Here's how the part is built. I have some questions about the finished solid (model axes, mm). A direction names the side the tool comes from. Coordinates: 2 decimals unless noted, no trailing zeros. Order: outer loops, then holes, each group sorted by start corner. A loop starts at its lowest first (then second) coordinate and runs counter-clockwise, first axis right, second up.
```python
from build123d import *

# Parameters (mm, degrees)
SKETCH1_W           = 12.25
SKETCH1_H           = 14.6
BOSS_EXTRUDE1_DEPTH = 13.13
CUT_EXTRUDE1_DEPTH  = 12.07
SKETCH4_W           = 10.22
SKETCH4_H           = 1.85
CUT_EXTRUDE3_DEPTH  = 10.5
CUT_EXTRUDE4_REACH  = 18.224
SKETCH5_W           = 0.518
SKETCH5_H           = 6.3
SKETCH6_W           = 9.9
SKETCH6_H           = 3.6
CUT_EXTRUDE5_DEPTH  = 1.9
SKETCH10_W          = 5.64
SKETCH10_H          = 2.85
CUT_EXTRUDE7_DEPTH  = 2.13
SKETCH11_W          = 9.9
SKETCH11_H          = 0.75
CUT_EXTRUDE8_DEPTH  = 15.728154161
SKETCH12_R          = 1
BOSS_EXTRUDE2_DEPTH = 2.9
FILLET1_R           = 0.25
SKETCH15_W          = 0.5
SKETCH15_H          = 0.5
BOSS_EXTRUDE3_DEPTH = 3.7
CHAMFER1_SIZE       = 0.05
SKETCH16_W          = 9.9
SKETCH16_H          = 0.6
BOSS_EXTRUDE4_DEPTH = 0.75
SKETCH17_W          = 0.518
SKETCH17_H          = 6.3
SKETCH17_W_2        = 10.25
SKETCH17_H_2        = 1.85
BOSS_EXTRUDE5_DEPTH = 2
SKETCH18_W          = 1.15
SKETCH18_H          = 10.25
BOSS_EXTRUDE6_DEPTH = 1


with BuildPart() as part:
    # Sketch1 → Boss-Extrude1 (new body)
    with BuildSketch(Plane.XY):
        Rectangle(SKETCH1_W, SKETCH1_H)
    extrude(amount=BOSS_EXTRUDE1_DEPTH)

    # Sketch2 → Cut-Extrude1 (cut)
    with BuildSketch(Plane.XY.offset(13.13)):
        Polygon((3.28, 3.2), (3.28, 4.75), (1.915, 4.75), (1.915, 6.55), (-1.915, 6.55), (-1.915, 4.75), (-3.28, 4.75), (-3.28, 3.2), (-4.95, 3.2), (-4.95, -3.7), (4.95, -3.7), (4.95, 3.2), align=None)
    extrude(amount=-CUT_EXTRUDE1_DEPTH, mode=Mode.SUBTRACT)

    # Sketch4 → Cut-Extrude3 (cut)
    with BuildSketch(Plane(origin=(0, 0, 0), x_dir=(-1, 0, 0), z_dir=(0, 0, -1))):
        with Locations((0, 5.375)):
            Rectangle(SKETCH4_W, SKETCH4_H)
    extrude(amount=-CUT_EXTRUDE3_DEPTH, mode=Mode.SUBTRACT)

    # Sketch5 → Cut-Extrude4 (cut, up to next)
    with BuildSketch(Plane(origin=(0, 0, 0), x_dir=(-1, 0, 0), z_dir=(0, 0, -1)), mode=Mode.PRIVATE) as cut_extrude4_sk1:
        with Locations((-1.555, -0.4)):
            Rectangle(SKETCH5_W, SKETCH5_H)
    cut_extrude4_tool1 = extrude(cut_extrude4_sk1.sketch, amount=-CUT_EXTRUDE4_REACH, mode=Mode.PRIVATE) & part.part
    # Sketch5 → Cut-Extrude4 (cut, up to next)
    with BuildSketch(Plane(origin=(0, 0, 0), x_dir=(-1, 0, 0), z_dir=(0, 0, -1)), mode=Mode.PRIVATE) as cut_extrude4_sk2:
        with Locations((-0.519, -0.4)):
            Rectangle(SKETCH5_W, SKETCH5_H)
    cut_extrude4_tool2 = extrude(cut_extrude4_sk2.sketch, amount=-CUT_EXTRUDE4_REACH, mode=Mode.PRIVATE) & part.part
    # Sketch5 → Cut-Extrude4 (cut, up to next)
    with BuildSketch(Plane(origin=(0, 0, 0), x_dir=(-1, 0, 0), z_dir=(0, 0, -1)), mode=Mode.PRIVATE) as cut_extrude4_sk3:
        with Locations((0.519, -0.4)):
            Rectangle(SKETCH5_W, SKETCH5_H)
    cut_extrude4_tool3 = extrude(cut_extrude4_sk3.sketch, amount=-CUT_EXTRUDE4_REACH, mode=Mode.PRIVATE) & part.part
    # Sketch5 → Cut-Extrude4 (cut, up to next)
    with BuildSketch(Plane(origin=(0, 0, 0), x_dir=(-1, 0, 0), z_dir=(0, 0, -1)), mode=Mode.PRIVATE) as cut_extrude4_sk4:
        with Locations((1.555, -0.4)):
            Rectangle(SKETCH5_W, SKETCH5_H)
    cut_extrude4_tool4 = extrude(cut_extrude4_sk4.sketch, amount=-CUT_EXTRUDE4_REACH, mode=Mode.PRIVATE) & part.part
    add(cut_extrude4_tool1.solids().sort_by_distance((1.555, -0.4, 0))[0], mode=Mode.SUBTRACT)
    add(cut_extrude4_tool2.solids().sort_by_distance((0.519, -0.4, 0))[0], mode=Mode.SUBTRACT)
    add(cut_extrude4_tool3.solids().sort_by_distance((-0.519, -0.4, 0))[0], mode=Mode.SUBTRACT)
    add(cut_extrude4_tool4.solids().sort_by_distance((-1.555, -0.4, 0))[0], mode=Mode.SUBTRACT)

    # Sketch6 → Cut-Extrude5 (cut)
    with BuildSketch(Plane.XY.offset(13.13)):
        with Locations((0, -5.5)):
            Rectangle(SKETCH6_W, SKETCH6_H)
    extrude(amount=-CUT_EXTRUDE5_DEPTH, mode=Mode.SUBTRACT)

    # Sketch10 → Cut-Extrude7 (cut)
    with BuildSketch(Plane.XY.offset(11.23)):
        with Locations((0, -5.125)):
            Rectangle(SKETCH10_W, SKETCH10_H)
    extrude(amount=-CUT_EXTRUDE7_DEPTH, mode=Mode.SUBTRACT)

    # Sketch11 → Cut-Extrude8 (cut, through all)
    with BuildSketch(Plane.XY.offset(11.23)):
        with Locations((0, -6.925)):
            Rectangle(SKETCH11_W, SKETCH11_H)
    extrude(amount=-CUT_EXTRUDE8_DEPTH, mode=Mode.SUBTRACT)

    # Sketch12 → Boss-Extrude2 (add)
    with BuildSketch(Plane.XZ.offset(7.3)):
        with Locations(Location((-6.125, 7, 0), (0, 0, 270))):
            Circle(SKETCH12_R)
        with Locations(Location((6.125, 7, 0), (0, 0, 90))):
            Circle(SKETCH12_R)
    extrude(amount=BOSS_EXTRUDE2_DEPTH)

    # Sketch13 → Revolve1 (revolve)
    with BuildSketch(Plane(origin=(6.125, 0, 0), x_dir=(0, 0, -1), z_dir=(1, 0, 0))):
        with BuildLine():
            Line((-7, -6.3), (-7, -7.3))
            Line((-7, -7.3), (-8, -7.3))
            ThreePointArc((-8, -7.3), (-7.707106781, -6.592893219), (-7, -6.3))
        make_face()
    revolve(axis=Axis((6.125, -6.3, 7), (0, -1, 0)))

    # Sketch14 → Revolve2 (revolve)
    with BuildSketch(Plane.ZY.offset(6.125)):
        with BuildLine():
            Line((7, -6.3), (7, -7.3))
            Line((7, -7.3), (6, -7.3))
            ThreePointArc((6, -7.3), (6.292893219, -6.592893219), (7, -6.3))
        make_face()
    revolve(axis=Axis((-6.125, -6.3, 7), (0, -1, 0)))

    # Fillet1
    fillet1_edges = [part.edges().sort_by_distance(p)[0] for p in [
        (-6.125, -10.2, 8),
        (6.125, -10.2, 6),
    ]]
    fillet(fillet1_edges, radius=FILLET1_R)

    # Sketch15 → Boss-Extrude3 (add)
    with BuildSketch(Plane.XZ.offset(6.55)):
        with Locations((-0.5, 4.5)):
            Rectangle(SKETCH15_W, SKETCH15_H)
        with Locations((-1.5, 2)):
            Rectangle(SKETCH15_W, SKETCH15_H)
        with Locations((0.5, 2)):
            Rectangle(SKETCH15_W, SKETCH15_H)
        with Locations((1.5, 4.5)):
            Rectangle(SKETCH15_W, SKETCH15_H)
    extrude(amount=BOSS_EXTRUDE3_DEPTH)

    # Chamfer1
    chamfer1_edges = [part.edges().sort_by_distance(p)[0] for p in [
        (-0.25, -10.25, 4.5),
        (-0.5, -10.25, 4.75),
        (-0.75, -10.25, 4.5),
        (-0.5, -10.25, 4.25),
        (-1.25, -10.25, 2),
        (-1.5, -10.25, 2.25),
        (-1.75, -10.25, 2),
        (-1.5, -10.25, 1.75),
        (0.75, -10.25, 2),
        (0.5, -10.25, 2.25),
        (0.25, -10.25, 2),
        (0.5, -10.25, 1.75),
        (1.75, -10.25, 4.5),
        (1.5, -10.25, 4.75),
        (1.25, -10.25, 4.5),
        (1.5, -10.25, 4.25),
    ]]
    chamfer(chamfer1_edges, length=CHAMFER1_SIZE)

    # Sketch16 → Boss-Extrude4 (add)
    with BuildSketch(Plane.XZ.offset(6.55)):
        with Locations((0, 7)):
            Rectangle(SKETCH16_W, SKETCH16_H)
    extrude(amount=BOSS_EXTRUDE4_DEPTH)

    # Sketch17 → Boss-Extrude5 (add)
    with BuildSketch(Plane(origin=(0, 0, 0), x_dir=(-1, 0, 0), z_dir=(0, 0, -1))):
        Polygon((-6.125, 7.3), (6.125, 7.3), (6.125, -7.3), (5.125, -7.3), (5.125, -4.3), (-5.125, -4.3), (-5.125, -7.3), (-6.125, -7.3), align=None)
        with Locations((-1.555, -0.4)):
            Rectangle(SKETCH17_W, SKETCH17_H, mode=Mode.SUBTRACT)
        with Locations((-0.519, -0.4)):
            Rectangle(SKETCH17_W, SKETCH17_H, mode=Mode.SUBTRACT)
        with Locations((0.519, -0.4)):
            Rectangle(SKETCH17_W, SKETCH17_H, mode=Mode.SUBTRACT)
        with Locations((1.555, -0.4)):
            Rectangle(SKETCH17_W, SKETCH17_H, mode=Mode.SUBTRACT)
        with Locations((0, 5.375)):
            Rectangle(SKETCH17_W_2, SKETCH17_H_2, mode=Mode.SUBTRACT)
    extrude(amount=BOSS_EXTRUDE5_DEPTH)

    # Sketch18 → Boss-Extrude6 (add)
    with BuildSketch(Plane(origin=(6.125, 0, 0), x_dir=(0, 0, -1), z_dir=(1, 0, 0))):
        with Locations((-10.305, 0.975)):
            Rectangle(SKETCH18_W, SKETCH18_H)
    boss_extrude6 = extrude(amount=BOSS_EXTRUDE6_DEPTH)

    # Mirror1: Boss-Extrude6 across plane
    add(boss_extrude6.mirror(Plane(origin=(0, 0, 0), x_dir=(0, 0, 1), z_dir=(1, 0, 0))))


solid = part.part
```
Q1. I need wall thicknesses on L1, parallel to Y at x = 4.75, z = 9.75; L2, parallel to X at y = 0.25, z = 0 (3 decimals); L3, parallel to Y at x = 0.75, z = 2.5. Which ranges of each line are inside material? Lowest first, please.
Q2. We'd pull the mould along X, two halves only. Please class faces 1 (the flat face through (-1.814, 0, 0)), 2 (the flat face through (7.125, 1, 10)), 3 (the flat face through (4, 3.2, 7)), 4 (the flat face through (-6.6, 0.9, 9.73)): pulls with the +X half, pulls with the -X half, needs draft (parallel to the pull), parting line crosses it, or undercut.
Q3. For faces 5 (the flat face through (-0.778, 0, 0)), 6 (the flat face through (-5.125, 5, -1)), 7 (the flat face through (-2.82, -5, 10)), 8 (the flat face through (0, 6.55, 7)), 9 (the flat face through (6.6, 0.9, 10.88)), which set-ups out of +Z, -Z, +X, -X, +Y, -Y let a thin tool reach every point of the face, with its end or its side?
Q4. Will these pins go through, and if not, where does the flat tip stop? pin 1 (2.5 mm diameter, centred on x = 1.5, y = 0, fed in from +Z); pin 2 (1.5 mm diameter, centred on y = 6, z = 6.5, fed in from +X) (3 decimals); pin 3 (5 mm diameter, centred on x = -5, z = 6.5, fed in from -Y).
Q5. If we section it at B-B on y = -3.25: Give the number of separate pieces and of enclosed holes in the cut face, then the cut area to 3 significant figures.
Q6. If we section it at A-A on x = -2.25: Write out the boundary of the cut face in (y, z), then the cut area to 3 significant figures.
Reply:
1. L1: y = -6.55 to -3.7, 3.2 to 4.45, 6.3 to 7.3
1. L2: x = -6.125 to -1.814, -1.296 to -0.778, -0.26 to 0.26, 0.778 to 1.296, 1.814 to 6.125
1. L3: y = -6.55 to -3.7, 6.55 to 7.3
2. face 1: undercut
2. face 2: pulls with the +X half
2. face 3: undercut
2. face 4: needs draft
3. face 5: +Z, -Z
3. face 6: -Z
3. face 7: +Z, -Y
3. face 8: +Z
3. face 9: +Z, +X, +Y, -Y
4. pin 1: stops at z = 1.06
4. pin 2: stops at x = 6.125
4. pin 3: stops at y = -10.2
5. separate pieces: 5
5. enclosed holes: 0
5. area: 61.8 mm2
6. outline: (-7.3, 6.7) - (-6.55, 6.7) - (-6.55, 0) - (-4.3, 0) - (-4.3, -2) - (4.45, -2) - (4.45, 1.06) - (-3.7, 1.06) - (-3.7, 9.1) - (-6.55, 9.1) - (-6.55, 7.3) - (-7.3, 7.3) - close; (4.75, 10.5) - (6.3, 10.5) - (6.3, -2) - (7.3, -2) - (7.3, 13.13) - (4.75, 13.13) - close
6. area: 71.7 mm2
